Model file for the job. Use its own axes, mm. A direction names the side the tool comes from. Give positions to 0.01 mm unless a question says otherwise; leave off trailing zeros. Write each loop counter-clockwise with the first axis right and the second up, starting at its lowest first coordinate (ties: lowest second). Pieces come first, ordered by that corner, then holes. Notation, with made-up numbers: (-20.75, 51) - (28.25, 51) arc R28 cw to (28.25, 70) - close; hole circle Ø6 at (-13.75, 89.25). An arc over 180 degrees is marked (long way). Use CSV: the item, a comma, the result in double quotes.
from build123d import *

# Parameters (mm, degrees)
F0_R     = 2.5
F0_R_2   = 7.144
F1_DEPTH = 6.35
F2_W     = 6.35
F2_H     = 38
F3_DEPTH = 37.876
F5_D     = 4
F5_DEPTH = 12
F5_TIP   = 1.2017212381
F7_D     = 4
F7_DEPTH = 12
F7_TIP   = 1.2017212381


with BuildPart() as f1:
    # F0 (on Right) → F1 (new body)
    with BuildSketch(Plane.YZ):
        with BuildLine():
            ThreePointArc((17.8751346366, -25.0354456965), (12.8773903734, -19.5640491806), (14.5155336292, -12.3370086917))
            ThreePointArc((14.5155336292, -12.3370086917), (9.7791608288, 16.348410121), (-17.735210007, 6.9544824399))
            ThreePointArc((-17.735210007, 6.9544824399), (-20.675525796, 3.2657587243), (-25.1830672278, 1.875))
            Line((-25.1830672278, 1.875), (-127.076, 1.875))
            Line((-127.076, 1.875), (-127.076, -4.475))
            Line((-127.076, -4.475), (-93.076, -4.475))
            ThreePointArc((-93.076, -4.475), (-90.2475728753, -5.6465728753), (-89.076, -8.475))
            Line((-89.076, -8.475), (-89.076, -22.475))
            ThreePointArc((-89.076, -22.475), (-90.2475728753, -25.3034271247), (-93.076, -26.475))
            Line((-93.076, -26.475), (-127.076, -26.475))
            Line((-127.076, -26.475), (-127.076, -32.825))
            Line((-127.076, -32.825), (-40.201, -32.825))
            Line((-40.201, -32.825), (-40.201, -36))
            Line((-40.201, -36), (48, -36))
            Line((48, -36), (17.8751346366, -25.0354456965))
        make_face()
        with BuildLine():
            ThreePointArc((-82.726, -8.475), (-81.5544271247, -5.6465728753), (-78.726, -4.475))
            Line((-78.726, -4.475), (-26.726, -4.475))
            ThreePointArc((-26.726, -4.475), (-23.8975728753, -5.6465728753), (-22.726, -8.475))
            Line((-22.726, -8.475), (-22.726, -22.475))
            ThreePointArc((-22.726, -22.475), (-23.8975728753, -25.3034271247), (-26.726, -26.475))
            Line((-26.726, -26.475), (-78.726, -26.475))
            ThreePointArc((-78.726, -26.475), (-81.5544271247, -25.3034271247), (-82.726, -22.475))
            Line((-82.726, -22.475), (-82.726, -8.475))
        make_face(mode=Mode.SUBTRACT)
        with Locations((0, -12.7)):
            Circle(F0_R, mode=Mode.SUBTRACT)
        with Locations((-12.7, 0)):
            Circle(F0_R, mode=Mode.SUBTRACT)
        Circle(F0_R_2, mode=Mode.SUBTRACT)
        with Locations((12.7, 0)):
            Circle(F0_R, mode=Mode.SUBTRACT)
        with Locations((0, 12.7)):
            Circle(F0_R, mode=Mode.SUBTRACT)
    extrude(amount=F1_DEPTH)

    # F2 (on face) → F3 (cut, through all)
    with BuildSketch(Plane.XY.offset(1.875)):
        with Locations((3.175, -108.076)):
            Rectangle(F2_W, F2_H)
    extrude(amount=-F3_DEPTH, mode=Mode.SUBTRACT)

    # F5
    with Locations(Plane.XY.offset(1.875)):
        with Locations((3.175, -83.076), (3.175, -47.076)):
            Hole(F5_D / 2, depth=F5_DEPTH)
            with Locations((0, 0, -(F5_DEPTH + F5_TIP / 2))):  # 118° drill point
                Cone(0, F5_D / 2, F5_TIP, mode=Mode.SUBTRACT)

    # F7
    with Locations(Plane(origin=(0, 0, -32.825), x_dir=(1, 0, 0), z_dir=(0, 0, -1))):
        with Locations((3.175, 83.076), (3.175, 47.076)):
            Hole(F7_D / 2, depth=F7_DEPTH)
            with Locations((0, 0, -(F7_DEPTH + F7_TIP / 2))):  # 118° drill point
                Cone(0, F7_D / 2, F7_TIP, mode=Mode.SUBTRACT)


solid = f1.part
(1) 3-axis set-ups, long thin cutter, end or side, ignore diameter. For faces 1 (the face through (3.44, -85.06, -28.07)), 2 (the face through (3, -57, 1.875)), 3 (the face through (3.61, -85.03, -2.88)), 4 (the face through (3.131, -23.929, -5.616)): which of +Z, -Z, +X, -X, +Y, -Y reach the whole face in a straight line?
Checked values:
face 1,"-Z"
face 2,"+Z, +X, -X, -Y"
face 3,"+Z"
face 4,"+X, -X"
(2) Saw through at B-B, the plane z = 0. List the corners of the cut face in (x, y) (3 decimals).
Checked values:
outline,"(0, -89.076) - (6.35, -89.076) - (6.35, -15.2) - (0, -15.2) - close; (0, -10.2) - (6.35, -10.2) - (6.35, -7.144) - (0, -7.144) - close; (0, 7.144) - (6.35, 7.144) - (6.35, 10.2) - (0, 10.2) - close; (0, 15.2) - (6.35, 15.2) - (6.35, 19.05) - (0, 19.05) - close; hole circle Ø4 at (3.175, -83.076); hole circle Ø4 at (3.175, -47.076)"
(3) Saw through at D-D, the plane z = 12.7. List the corners of the cut face in (x, y).
Checked values:
outline,"(0, -14.2) - (6.35, -14.2) - (6.35, -2.5) - (0, -2.5) - close; (0, 2.5) - (6.35, 2.5) - (6.35, 14.2) - (0, 14.2) - close"
(4) Wall check: probe 1 along Z at (x, y) = (2.5, 0); probe 2 along Z at (x, y) = (5.75, -51) (3 decimals); probe 3 along Y at (x, z) = (3, -3). Give the ranges that are in metal, low to high. Write a range as [from, to].
Checked values:
probe 1,"z = [-36, -15.2], [-10.2, -7.14], [7.14, 10.2], [15.2, 19.05]"
probe 2,"z = [-32.825, -26.475], [-4.475, 1.875]"
probe 3,"y = [-89.08, -85.07], [-81.08, -49.07], [-45.08, -6.48], [6.48, 18.81]"
(5) Saw through at C-C, the plane y = -68.5. List the corners of the cut face in (x, z) (3 decimals), then the cut area to 3 significant figures.
Checked values:
outline,"(0, -32.825) - (6.35, -32.825) - (6.35, -26.475) - (0, -26.475) - close; (0, -4.475) - (6.35, -4.475) - (6.35, 1.875) - (0, 1.875) - close"
area,"80.6 mm^2"
(6) Saw through at A-A, the plane y = 0. List the corners of the cut face in (x, z).
Checked values:
outline,"(0, -36) - (6.35, -36) - (6.35, -15.2) - (0, -15.2) - close; (0, -10.2) - (6.35, -10.2) - (6.35, -7.14) - (0, -7.14) - close; (0, 7.14) - (6.35, 7.14) - (6.35, 10.2) - (0, 10.2) - close; (0, 15.2) - (6.35, 15.2) - (6.35, 19.05) - (0, 19.05) - close"
(7) Flat gauge pins, fed straight in: P1, Ø3, axis at x = 3.5, y = -55.5, coming from the +Z side (3 decimals); P2, Ø3, axis at x = 4.5, y = -58, coming from the -Z side (3 decimals); P3, Ø1.9, axis at x = 3.5, z = -18, coming from the +Y side. Where does each tip first touch, or does it go through?
Checked values:
P1,"stops at z = 1.875"
P2,"stops at z = -32.825"
P3,"stops at y = 12.74"
(8) Pull direction Y, two halves, no side cores. Call faces 5 (the face through (6.35, -21, -14)), 6 (the face through (3, -89.076, -15)), 7 (the face through (3.131, 15.085, 0.751)), 8 (the face through (3.13, -0.33, -10.22)): released by +Y, released by -Y, zero draft, split by the parting line, or undercut.
Checked values:
face 5,"zero draft"
face 6,"released by -Y"
face 7,"undercut"
face 8,"undercut"
